Autodesk Inventor part; units mm, degrees
ref_plane "YZ Plane" through (0, 0, 0) normal (1, 0, 0) x (0, 1, 0)
ref_plane "XZ Plane" through (0, 0, 0) normal (0, 1, 0) x (-1, 0, 0)
ref_plane "XY Plane" through (0, 0, 0) normal (0, 0, 1) x (1, 0, 0)
sketch "Sketch1" plane through (0, 0, 0) normal (0, 1, 0) x (-1, 0, 0)
  circle A0 centre (0, 0) radius 15
  circle A1 centre (0, 0) radius 15.5
  dimension "d0" = 30
  dimension "d1" = 31
extrude "Extrusion1" add sketch "Sketch1" along normal blind 1000
sketch "Sketch2" plane through (0, 0, 0) normal (0, 0, 1) x (1, 0, 0)
  line L0 (0, 0) -> (0, 6)
  line L1 (0, 0) -> (6, 0) construction
  circle A0 centre (0, 6) radius 1.5
  line L2 (15.5, 1000) -> (-15.5, 1000)
  line L3 (0, 1000) -> (0, 994)
  circle A1 centre (0, 994) radius 1.5
  dimension "d4" = 6
  dimension "d5" = 90
  dimension "d6" = 3
  dimension "d7" = 6
  dimension "d8" = 3
extrude "Extrusion2" cut sketch "Sketch2" along normal mid plane 40
properties part number "30 mm tube"
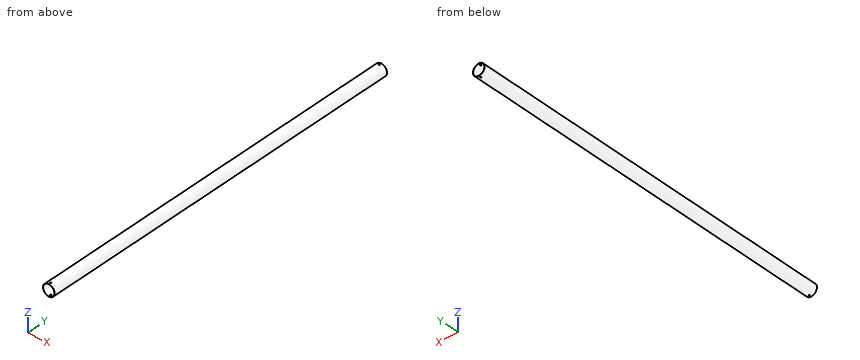
Verification items for the finished model (mm, model axes). Give positions to 0.01 mm unless a question says otherwise; leave off trailing zeros. Write each loop counter-clockwise with the first axis right and the second up, starting at its lowest first coordinate (ties: lowest second). Pieces come first, ordered by that corner, then holes. Notation, with made-up numbers: M -14.75,-39.5 L -0.75,-39.5 A17 ccw -0.75,-26.5 Z; hole C -19,53.25 d1. An arc over 180 degrees is marked long. One line per question, with ' | ' between items.
1) Section check B-B on y = 464. Enter the section's corners in (x, z).
Result:
outline: C 0,0 d31; hole C 0,0 d30
2) Thickness scan on line 1 along Y through (x, z) = (0, 15.15); line 2 along Z through (x, y) = (0, 258); line 3 along X through (y, z) = (926, 0.5). Record the ranges inside material, lowest first. Write a range as [from, to].
Result:
line 1: y = [0, 4.5], [7.5, 992.5], [995.5, 1000] | line 2: z = [-15.5, -15], [15, 15.5] | line 3: x = [-15.49, -14.99], [14.99, 15.49]
3) Section check A-A on z = 0. Enter the section's corners in (x, y), plus the area to 3 significant figures.
Result:
outline: M -15.5,0 L -15,0 L -15,1000 L -15.5,1000 Z; M 15,0 L 15.5,0 L 15.5,1000 L 15,1000 Z | area: 1,000 mm2
4) Gauge pin test, flat ends, axial feed: pin 1 Ø10 at (x, y) = (11.5, 122) entering from -Z; pin 2 Ø3 at (y, z) = (443, -4) entering from +X; pin 3 Ø4 at (y, z) = (797, 2.5) entering from +X. Record the tip position at first contact, or that the pin passes through.
Result:
pin 1: stops at z = -14.07 | pin 2: stops at x = 15.3 | pin 3: stops at x = 15.49
